Answer from the drawing. Dimensions are ordinates in mm from the lowest x, y and z of the part. Give positions to 0.01 mm unless a question says otherwise; leave off trailing zeros. Loops run counter-clockwise (first coordinate to the right, second up) from the corner with the lowest first, then second, coordinate; pieces in that order, holes last.
Item 1: Consider line 1 along Y through (x, z) = (19, 0.45); line 2 along Y through (x, z) = (7, 0.25); line 3 along Y through (x, z) = (13, 0.5). Determine where each line is inside the solid, lowest interval first.
Item 2: This flat-tipped pin is pushed along its axis until it touches: pin 1 Ø6 at (x, y) = (9, 13) entering from +Z. Where does it stop, or does it pass through?
Item 3: Section C-C, the plane x = 13 is taken. Give the vertices of the cut face in (y, z), and give its area (3 significant figures).
Item 4: Section D-D, the plane y = 7 is taken. Give the vertices of the cut face in (x, z), and give its area (3 significant figures).
Item 5: Section B-B, the plane z = 0.55 is taken. Give the vertices of the cut face in (x, y).
Item 6: Section A-A, the plane y = 13 is taken. Give the vertices of the cut face in (x, z), and give its area (3 significant figures).
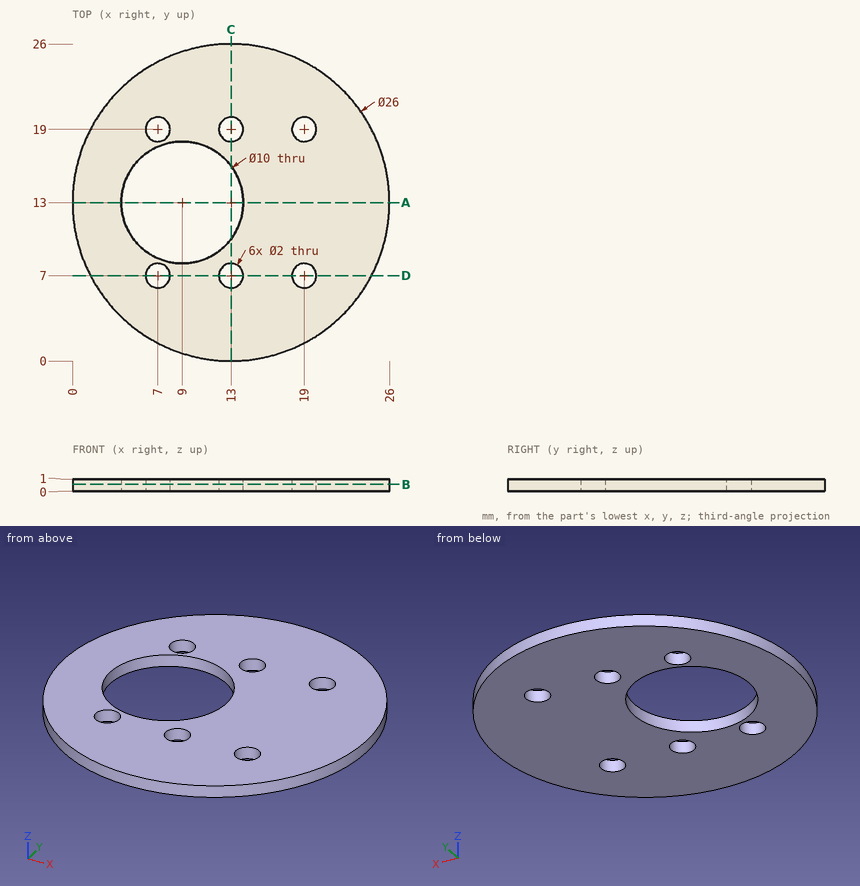
Worked answers:
1. line 1: y = 1.47 to 6, 8 to 18, 20 to 24.53
1. line 2: y = 1.47 to 6, 8 to 8.42, 17.58 to 18, 20 to 24.53
1. line 3: y = 0 to 6, 8 to 10, 16 to 18, 20 to 26
2. pin 1: passes through
3. outline: (0, 0) - (6, 0) - (6, 1) - (0, 1) - close; (8, 0) - (10, 0) - (10, 1) - (8, 1) - close; (16, 0) - (18, 0) - (18, 1) - (16, 1) - close; (20, 0) - (26, 0) - (26, 1) - (20, 1) - close
3. area: 16.0 mm2
4. outline: (1.47, 0) - (6, 0) - (6, 1) - (1.47, 1) - close; (8, 0) - (12, 0) - (12, 1) - (8, 1) - close; (14, 0) - (18, 0) - (18, 1) - (14, 1) - close; (20, 0) - (24.53, 0) - (24.53, 1) - (20, 1) - close
4. area: 17.1 mm2
5. outline: circle Ø26 at (13, 13); hole circle Ø10 at (9, 13); hole circle Ø2 at (7, 7); hole circle Ø2 at (7, 19); hole circle Ø2 at (13, 7); hole circle Ø2 at (13, 19); hole circle Ø2 at (19, 7); hole circle Ø2 at (19, 19)
6. outline: (0, 0) - (4, 0) - (4, 1) - (0, 1) - close; (14, 0) - (26, 0) - (26, 1) - (14, 1) - close
6. area: 16.0 mm2
